For this review, take the finished solid that the model builds, in its own axes (mm). A direction names the side the tool comes from. Give positions to 0.01 mm unless a question says otherwise; leave off trailing zeros. Loops run counter-clockwise (first coordinate to the right, second up) from the corner with the lowest first, then second, coordinate; pieces in that order, holes last. Notation, with made-up numbers: (42.5, -8) - (46.5, -8) arc R16 ccw to (46.5, 11) - close; hole circle Ø1 at (18.5, 10.25). An arc over 180 degrees is marked (long way). Put each result on its own line as item: value.
from build123d import *

# Parameters (mm, degrees)
IZIM1_R                          = 20
IZIM1_R_2                        = 13
Y_KSEKLIK_EKSTR_ZYON1_DEPTH      = 25
IZIM2_W                          = 75
IZIM2_H                          = 25
Y_KSEKLIK_EKSTR_ZYON3_DEPTH      = 55.415897
Y_KSEKLIK_EKSTR_ZYON3_DEPTH_BACK = 56.584103
KES_EKSTR_ZYON1_DEPTH            = 76
IZIM5_R                          = 10
KES_EKSTR_ZYON2_DEPTH            = 26
KES_EKSTR_ZYON3_DEPTH            = 26
IZIM1_7_R                        = 20
IZIM1_7_R_2                      = 13
Y_KSEKLIK_EKSTR_ZYON6_DEPTH      = 50


with BuildPart() as part:
    # Çizim1 → Yükseklik-Ekstrüzyon1 (new body)
    with BuildSketch(Plane.XY):
        with BuildLine():
            Line((20.815714115, 93.071898447), (55.415896847, -40.357088497))
            Line((55.415896847, -40.357088497), (-56.584103153, -40.357088497))
            Line((-56.584103153, -40.357088497), (-21.983920421, 93.071898447))
            ThreePointArc((-21.983920421, 93.071898447), (-0.584103153, 107.642911503), (20.815714115, 93.071898447))
        make_face()
        with Locations((-0.584103153, 84.642911503)):
            Circle(IZIM1_R, mode=Mode.SUBTRACT)
        with Locations((-0.584103153, 84.642911503)):
            Circle(IZIM1_R)
        with Locations((-0.584103153, 84.642911503)):
            Circle(IZIM1_R_2, mode=Mode.SUBTRACT)
    extrude(amount=Y_KSEKLIK_EKSTR_ZYON1_DEPTH)

    # Çizim2 → Yükseklik-Ekstrüzyon3 (add, two sides)
    with BuildSketch(Plane(origin=(0, 0, 0), x_dir=(0, 0, -1), z_dir=(1, 0, 0))) as y_kseklik_ekstr_zyon3_sk:
        with Locations((-37.5, -52.857088497)):
            Rectangle(IZIM2_W, IZIM2_H)
    extrude(amount=Y_KSEKLIK_EKSTR_ZYON3_DEPTH)
    extrude(y_kseklik_ekstr_zyon3_sk.sketch, amount=-Y_KSEKLIK_EKSTR_ZYON3_DEPTH_BACK)

    # Çizim3 → Kes-Ekstrüzyon1 (cut, through all)
    with BuildSketch(Plane.XY.offset(75)):
        Polygon((-10.584103153, -65.357088497), (-0.584103153, -55.357088497), (9.415896847, -65.357088497), align=None)
    extrude(amount=-KES_EKSTR_ZYON1_DEPTH, mode=Mode.SUBTRACT)

    # Çizim5 → Kes-Ekstrüzyon2 (cut, through all)
    with BuildSketch(Plane(origin=(0, -40.357088497, 0), x_dir=(1, 0, 0), z_dir=(0, 1, 0))):
        with Locations((-0.584103153, -50)):
            Circle(IZIM5_R)
    extrude(amount=-KES_EKSTR_ZYON2_DEPTH, mode=Mode.SUBTRACT)

    # Çizim8 → Kes-Ekstrüzyon3 (cut, through all)
    with BuildSketch(Plane.XY.offset(25)):
        with BuildLine():
            Line((-19.943777352, 21.2621788), (-30.864373198, -20.851010365))
            ThreePointArc((-30.864373198, -20.851010365), (-29.801809113, -26.028840886), (-25.056470938, -28.357088497))
            Line((-25.056470938, -28.357088497), (23.888264632, -28.357088497))
            ThreePointArc((23.888264632, -28.357088497), (28.633602807, -26.028840886), (29.696166892, -20.851010365))
            Line((29.696166892, -20.851010365), (18.775571046, 21.2621788))
            ThreePointArc((18.775571046, 21.2621788), (-0.584103153, 36.241918358), (-19.943777352, 21.2621788))
        make_face()
    extrude(amount=-KES_EKSTR_ZYON3_DEPTH, mode=Mode.SUBTRACT)

    # Çizim1<7> → Yükseklik-Ekstrüzyon6 (add)
    with BuildSketch(Plane.XY):
        with Locations((-0.584103153, 84.642911503)):
            Circle(IZIM1_7_R)
        with Locations((-0.584103153, 84.642911503)):
            Circle(IZIM1_7_R_2, mode=Mode.SUBTRACT)
    extrude(amount=Y_KSEKLIK_EKSTR_ZYON6_DEPTH)


solid = part.part
1) Take a section at D-D on x = 16.5. State the section outline as (y, z) points.
Geometry check:
outline: (-65.36, 0) - (-28.36, 0) - (-28.36, 25) - (-40.36, 25) - (-40.36, 75) - (-65.36, 75) - close; (26.64, 0) - (100.04, 0) - (100.04, 25) - (95.04, 25) - (95.04, 50) - (74.24, 50) - (74.24, 25) - (26.64, 25) - close
2) Draft analysis for pull direction Y (two halves, no side actions). For faces 5 (the face through (-12, 35, 25)), 6 (the face through (33, -65.357, 38)), 7 (the face through (-25.328, 0.5, 12.675)), 8 (the face through (0, -53, 75)), state which applies: pulls with the +Y half, pulls with the -Y half, needs draft (parallel to the pull), parting line crosses it, or undercut.
Geometry check:
face 5: undercut
face 6: pulls with the -Y half
face 7: undercut
face 8: needs draft
3) Wall thickness on line 1 (X direction, y = -50.75, z = 50); line 2 (X direction, y = -49, z = 58.5); line 3 (Z direction, x = -17, y = 56): over which ranges is each line inside the solid? List them lowest first.
Geometry check:
line 1: x = -56.58 to -10.58, 9.42 to 55.42
line 2: x = -56.58 to -5.85, 4.68 to 55.42
line 3: z = 0 to 25
4) Take a section at C-C on x = 1.5. State the section outline as (y, z) points, and give its area (3 significant figures).
Geometry check:
outline: (-57.44, 0) - (-28.36, 0) - (-28.36, 25) - (-40.36, 25) - (-40.36, 40.22) - (-57.44, 40.22) - close; (-57.44, 59.78) - (-40.36, 59.78) - (-40.36, 75) - (-57.44, 75) - close; (36.13, 0) - (71.81, 0) - (71.81, 50) - (64.75, 50) - (64.75, 25) - (36.13, 25) - close; (97.47, 0) - (107.55, 0) - (107.55, 25) - (104.53, 25) - (104.53, 50) - (97.47, 50) - close
area: 2,740 mm²
5) Take a section at B-B on y = -44. State the section outline as (x, z) points.
Geometry check:
outline: (-56.58, 0) - (55.42, 0) - (55.42, 75) - (-56.58, 75) - close; hole circle Ø20 at (-0.58, 50)
6) Insertion check: pin 1 Ø1 at (y, z) = (30, 24) entering from -X; pin 2 Ø25 at (x, z) = (-6, 55.5) entering from +Y; pin 3 Ø4 at (x, y) = (32, 24.5) entering from +Z. Each pin has a flat end and moves straight along its axis. Give the tip position at first contact, or say it passes through.
Geometry check:
pin 1: stops at x = -38.47
pin 2: stops at y = 104.64
pin 3: stops at z = 25
7) Take a section at A-A on z = 29. State the section outline as (x, y) points, and give its area (3 significant figures).
Geometry check:
outline: (-56.58, -65.36) - (-10.58, -65.36) - (-0.58, -55.36) - (9.42, -65.36) - (55.42, -65.36) - (55.42, -40.36) - (-56.58, -40.36) - close; circle Ø40 at (-0.58, 84.64); hole circle Ø26 at (-0.58, 84.64)
area: 3,430 mm²
8) For faces 1 (the face through (-3.188, 104.473, 37.325)), 2 (the face through (12, 80, 50)), 3 (the face through (4.35, -60.29, 65.45)), 4 (the face through (24.312, -0.089, 12.675)), list the 3-axis set-ups (+Z, -Z, +X, -X, +Y, -Y) from which the entire face can be reached by the end or side of a thin tool; tool diameter is ignored.
Geometry check:
face 1: +Z
face 2: +Z, +X, -X, +Y
face 3: +Z, -Z, -Y
face 4: +Z, -Z
